Build history of the part. All positions in model axes, mm. A direction names the side the tool comes from. Round coordinates to 2 decimals unless told otherwise and drop trailing zeros. Write each loop counter-clockwise with the first axis right and the second up, starting at its lowest first coordinate (ties: lowest second). Pieces come first, ordered by that corner, then holes. Notation, with made-up numbers: (78.5, -17.5) - (104.5, -17.5) arc R17 cw to (104.5, -4.5) - close; hole circle Ø11 at (44.5, 26). An arc over 180 degrees is marked (long way). Write each question's results on one line, items separated by ' | '.
Autodesk Inventor part; units mm, degrees
ref_plane "YZ Plane" through (0, 0, 0) normal (1, 0, 0) x (0, 1, 0)
ref_plane "XZ Plane" through (0, 0, 0) normal (0, 1, 0) x (-1, 0, 0)
ref_plane "XY Plane" through (0, 0, 0) normal (0, 0, 1) x (1, 0, 0)
sketch "Sketch1" plane through (0, 0, 0) normal (0, 0, 1) x (1, 0, 0)
  line L0 (0, 0) -> (-2.5, 0)
  line L1 (-2.5, 0) -> (-2.5, 3)
  line L2 (-2.5, 3) -> (-3.5, 3)
  line L3 (-3.5, 3) -> (-3.5, 4.5)
  line L4 (0, 0) -> (0, 20)
  line L5 (0, 20) -> (0, 13)
  arc A0 (0, 20) -> (-4.0129, 7.2645) centre (0, 13) ccw
  line L6 (-3.5, 4.5) -> (-3.4274, 4.6257)
  line L7 (-3.5, 4.5) -> (-1.2818, 4.5) construction
  arc A1 (-3.4274, 4.6257) -> (-4.0129, 7.2645) centre (-5.1595, 5.6257) ccw
  point P0 (-2.3909, 6.421)
  dimension "d0" = 2.5
  dimension "d1" = 3
  dimension "d2" = 1
  dimension "d3" = 1.5
  dimension "d4" = 20
  dimension "d5" = 7
  dimension "d6" = 60
  dimension "d7" = 2
revolve "Revolution1" add sketch "Sketch1" angle 360 about axis through (0, 0, 0) along (0, 1, 0)
sketch "Sketch2" plane through (0, 0, 0) normal (0, -1, 0) x (1, 0, 0)
  circle A0 centre (0, 0) radius 2
  circle A1 centre (0, 0) radius 2.5
  line L0 (-2.5, 0.65) -> (2.5, 0.65)
  line L1 (2.5, 0.65) -> (2.5, -0.65)
  line L2 (2.5, -0.65) -> (-2.5, -0.65)
  line L3 (-2.5, -0.65) -> (-2.5, 0.65)
  line L4 (-2.5, 0.65) -> (2.5, -0.65) construction
  line L5 (2.5, 0.65) -> (-2.5, -0.65) construction
  line L6 (-0.65, 2.5) -> (-0.65, -2.5)
  line L7 (-0.65, -2.5) -> (0.65, -2.5)
  line L8 (0.65, -2.5) -> (0.65, 2.5)
  line L9 (0.65, 2.5) -> (-0.65, 2.5)
  circle A2 centre (0, 0) radius 2.5
  line L10 (-0.65, 2.5) -> (0.65, -2.5) construction
  line L11 (-0.65, -2.5) -> (0.65, 2.5) construction
  point P0 (0.65, -1.8914)
  point P1 (0.65, -2.414)
  point P2 (2.414, -0.65)
  point P3 (1.8914, -0.65)
  point P4 (0.65, 2.414)
  point P5 (0.65, 1.8914)
  point P6 (1.8914, 0.65)
  point P7 (2.414, 0.65)
  point P8 (-0.65, 1.8914)
  point P9 (-0.65, 2.414)
  point P10 (-2.414, 0.65)
  point P11 (-1.8914, 0.65)
  point P12 (-0.65, -2.414)
  point P13 (-0.65, -1.8914)
  point P14 (-1.8914, -0.65)
  point P15 (-2.414, -0.65)
  dimension "d9" = 4
  dimension "d10" = 5
  dimension "d11" = 1.3
  dimension "d12" = 1.3
extrude "Extrusion1" cut sketch "Sketch2" against normal blind 3 contours A0 L8 A1 L0 | L2 A1 L8 A0 | A0 L0 A1 L6 | L6 A1 L2 A0
properties part number "Ball"
(1) Slice it at B-B, the plane y = 5. Write the cut outline in (x, z), and give its area (3 significant figures).
Worked answers:
outline: circle Ø6.52 at (0, 0) | area: 33.4 mm2
(2) Tool access for faces 1 (the cylindrical face through (0, 1.5, 2.5)), 2 (the cylindrical face through (2.5, 1.5, 0)), 3 (the cylindrical face through (-3.233, 3.76, -1.341)), 4 (the cylindrical face through (1.41, 1.48, -1.42)), 5 (the cylindrical face through (-1.41, 1.48, 1.42)): list every direction of +Z, -Z, +X, -X, +Y, -Y with a clear straight run to the whole face (end or side of a thin tool).
Worked answers:
face 1: +Z, -Y | face 2: +X, -Y | face 3: -Y | face 4: -Z, +X, -Y | face 5: +Z, -X, -Y
(3) Drill centre lines: probe 1 along Z at (x, y) = (-2.25, 2); probe 2 along X at (y, z) = (16.5, -1.5). Where is each one in solid material? Low to high. Write a range as [from, to].
Worked answers:
probe 1: z = [-0.65, 0.65] | probe 2: x = [-5.87, 5.87]
(4) Slice it at A-A, the plane y = 2.5. Write the cut outline in (x, z).
Worked answers:
outline: (-2.41, -0.65) - (-1.89, -0.65) arc R2 ccw to (-0.65, -1.89) - (-0.65, -2.41) arc R2.5 ccw to (0.65, -2.41) - (0.65, -1.89) arc R2 ccw to (1.89, -0.65) - (2.41, -0.65) arc R2.5 ccw to (2.41, 0.65) - (1.89, 0.65) arc R2 ccw to (0.65, 1.89) - (0.65, 2.41) arc R2.5 ccw to (-0.65, 2.41) - (-0.65, 1.89) arc R2 ccw to (-1.89, 0.65) - (-2.41, 0.65) arc R2.5 ccw to start
(5) Flat gauge pins, fed straight in: pin 1 Ø2 at (y, z) = (9, -2.5) entering from +X; pin 2 Ø3 at (x, z) = (-2.5, 3.5) entering from +Y; pin 3 Ø2 at (x, y) = (3.5, 4.5) entering from -Z. Where does each tip first touch, or does it go through?
Worked answers:
pin 1: stops at x = 5.93 | pin 2: stops at y = 19.42 | pin 3: stops at z = -2.45
